```python
from build123d import *

# Parameters (mm, degrees)
SKETCH_1_W              = 20
SKETCH_1_H              = 340
EXTRUDE_1_DEPTH         = 800
HOLE_WIZARD_M12_1_D     = 10.2
HOLE_WIZARD_M12_1_DEPTH = 11.935610843
HOLE_WIZARD_M12_1_TIP   = 3.064389157
SKETCH_5_W              = 77.75
SKETCH_5_H              = 319.875
CUT_EXTRUDE_1_DEPTH     = 819.107572389
SKETCH_6_W              = 98
SKETCH_6_H              = 5
EXTRUDE_2_DEPTH         = 35


with BuildPart() as part:
    # 草图1 → 凸台-拉伸1 (new body)
    with BuildSketch(Plane.XY):
        Rectangle(SKETCH_1_W, SKETCH_1_H)
    extrude(amount=EXTRUDE_1_DEPTH)

    # M12 螺纹孔1
    with Locations(Plane(origin=(10, 0, 0), x_dir=(0, 0, -1), z_dir=(1, 0, 0))):
        with Locations((-529.599389894, -26.421356237), (-529.599389894, -146.421356237), (-604.599389894, -146.421356237), (-604.599389894, -26.421356237)):
            Hole(HOLE_WIZARD_M12_1_D / 2, depth=HOLE_WIZARD_M12_1_DEPTH)
            with Locations((0, 0, -(HOLE_WIZARD_M12_1_DEPTH + HOLE_WIZARD_M12_1_TIP / 2))):  # 118° drill point
                Cone(0, HOLE_WIZARD_M12_1_D / 2, HOLE_WIZARD_M12_1_TIP, mode=Mode.SUBTRACT)

    # 草图5 → 切除-拉伸1 (cut, through all)
    with BuildSketch(Plane(origin=(10, 0, 0), x_dir=(0, 0, -1), z_dir=(1, 0, 0))):
        with Locations((-38.875, 10.0625)):
            Rectangle(SKETCH_5_W, SKETCH_5_H)
    extrude(amount=-CUT_EXTRUDE_1_DEPTH, mode=Mode.SUBTRACT)

    # 草图6 → 凸台-拉伸2 (add)
    with BuildSketch(Plane(origin=(10, 0, 0), x_dir=(0, 0, -1), z_dir=(1, 0, 0))):
        with Locations((-126.75, -112.3)):
            Rectangle(SKETCH_6_W, SKETCH_6_H)
    extrude(amount=EXTRUDE_2_DEPTH)


solid = part.part
```
CAD build for the part. Positions are in the model's coordinates, mm. A direction names the side the tool comes from. Coordinates: 2 decimals unless noted, no trailing zeros. Loops run counter-clockwise (first coordinate to the right, second up) from the corner with the lowest first, then second, coordinate; pieces in that order, holes last. Notation, with made-up numbers: (36.5, 14) - (83.5, 14) arc R15 cw to (83.5, 35) - close; hole circle Ø2 at (-33, -31). An arc over 180 degrees is marked (long way). Return JSON: item names as keys, results as strings.
1. Drop flat-ended pins along their axis: pin 1 (3 mm diameter, centred on x = 6.5, y = 80.5, fed in from -Z); pin 2 (2 mm diameter, centred on y = 111.5, z = 546.5, fed in from +X); pin 3 (8 mm diameter, centred on y = -146.42, z = 529.6, fed in from +X). Give the stop position or say it passes through.
Result:
{"pin 1": "stops at z = 77.75", "pin 2": "stops at x = 10", "pin 3": "stops at x = -2.6"}
2. Band-saw the part on B-B (y = 57.5). Give the cut face in (x, z).
Result:
{"outline": "(-10, 77.75) - (10, 77.75) - (10, 800) - (-10, 800) - close"}
3. Probe L1, parallel to Z at x = 4, y = -12; L2, parallel to X at y = 101, z = 407.5; L3, parallel to Z at x = 6, y = -150.5. List the from-to ranges inside material, lowest first. Write a range as from..to.
Result:
{"L1": "z = 77.75..800", "L2": "x = -10..10", "L3": "z = 0..526.54, 532.66..601.54, 607.66..800"}
4. Band-saw the part on A-A (z = 88.5). Give the cut face in (x, y), and give its area (4 significant figures).
Result:
{"outline": "(-10, -170) - (10, -170) - (10, -114.8) - (45, -114.8) - (45, -109.8) - (10, -109.8) - (10, 170) - (-10, 170) - close", "area": "6,975 mm2"}
5. 3-axis set-ups, long thin cutter, end or side, ignore diameter. For faces 1 (the flat face through (27, -109.8, 127)), 2 (the flat face through (-10, -2, 394)), 3 (the flat face through (0, -149.875, 39)), 4 (the flat face through (27, -114.8, 127)), 5 (the flat face through (0, -170, 394)): which of +Z, -Z, +X, -X, +Y, -Y reach the whole face in a straight line?
Result:
{"face 1": "+Z, -Z, +X, +Y", "face 2": "+Z, -Z, -X, +Y, -Y", "face 3": "-Z, +X, -X, +Y", "face 4": "+Z, -Z, +X, -Y", "face 5": "+Z, -Z, +X, -X, -Y"}
6. Band-saw the part on C-C (x = 34). Give the cut face in (y, z), and give its area (3 significant figures).
Result:
{"outline": "(-114.8, 77.75) - (-109.8, 77.75) - (-109.8, 175.75) - (-114.8, 175.75) - close", "area": "490 mm2"}
